Geometry: final body of the model. Coordinates: model frame, mm. A direction names the side the tool comes from. Round coordinates to 2 decimals unless told otherwise and drop trailing zeros. Loops run counter-clockwise (first coordinate to the right, second up) from the corner with the lowest first, then second, coordinate; pieces in that order, holes last. Notation, with made-up numbers: (-31.5, 73) - (-21.5, 73) arc R19 cw to (-21.5, 88) - close; hole circle Ø1 at (2.25, -20). An arc over 180 degrees is marked (long way). Use CSV: the item, a comma, the result in double quotes.
from build123d import *

# Parameters (mm, degrees)
F0_W     = 304.8
F0_H     = 508
F1_DEPTH = 45.72
F3_W     = 267.97
F3_H     = 480.06
F4_DEPTH = 88.9
F5_R     = 88.9
F6_DEPTH = 6.35
F7_R     = 15.24
F8_DEPTH = 12.7


with BuildPart() as f1:
    # F0 (on Top) → F1 (new body)
    with BuildSketch(Plane.XY):
        with Locations((-4.550833, 30.915228)):
            Rectangle(F0_W, F0_H)
    extrude(amount=F1_DEPTH)

    # F3 (on face) → F4 (join)
    with BuildSketch(Plane(origin=(0, 0, 0), x_dir=(1, 0, 0), z_dir=(0, 0, -1))):
        with Locations((-4.550833, -30.915228)):
            Rectangle(F3_W, F3_H)
    extrude(amount=F4_DEPTH)

    # F5 (on face) → F6 (cut)
    with BuildSketch(Plane.XY.offset(45.72)):
        with Locations((0, 157.915228)):
            Circle(F5_R)
        with Locations((0, -45.284772)):
            Circle(F5_R)
    extrude(amount=-F6_DEPTH, mode=Mode.SUBTRACT)

    # F7 (on face) → F8 (join)
    with BuildSketch(Plane.XY.offset(45.72)):
        with Locations((-42.650833, -185.567364)):
            Circle(F7_R)
        with Locations((33.549167, -185.567364)):
            Circle(F7_R)
    extrude(amount=F8_DEPTH)


solid = f1.part
Item 1: Mould query, pull axis Y, two halves, no side actions, for faces 1 (the cylindrical face through (-70.548, -99.379, 42.589)), 2 (the flat face through (-138.536, 34, -44)), 3 (the flat face through (-7, 284.915, 23)). Classes: released by +Y, released by -Y, zero draft, split by the parting line, or undercut.
Final values:
face 1,"undercut"
face 2,"zero draft"
face 3,"released by +Y"
Item 2: Section A-A on y = 254.5. Return the cut outline in (x, z).
Final values:
outline,"(-156.95, 0) - (-138.54, 0) - (-138.54, -88.9) - (129.43, -88.9) - (129.43, 0) - (147.85, 0) - (147.85, 45.72) - (-156.95, 45.72) - close"
Item 3: Pin query (flat end, axial travel): P1, Ø1, axis at y = 61.5, z = -57.5, coming from the +X side; P2, Ø8, axis at y = 207, z = -1, coming from the -X side; P3, Ø12, axis at x = -65, y = 171.5, coming from the +Z side; P4, Ø12, axis at x = 113.5, z = -43, coming from the -Y side. Return the tip coordinate at first contact, or that it passes through.
Final values:
P1,"stops at x = 129.43"
P2,"stops at x = -156.95"
P3,"stops at z = 39.37"
P4,"stops at y = -209.11"
Item 4: Section D-D on x = -76. Return the cut outline in (y, z), plus the area to 3 significant figures.
Final values:
outline,"(-223.08, 0) - (-209.11, 0) - (-209.11, -88.9) - (270.95, -88.9) - (270.95, 0) - (284.92, 0) - (284.92, 45.72) - (204.04, 45.72) - (204.04, 39.37) - (111.79, 39.37) - (111.79, 45.72) - (0.84, 45.72) - (0.84, 39.37) - (-91.41, 39.37) - (-91.41, 45.72) - (-223.08, 45.72) - close"
area,"64,700 mm²"
Item 5: Section C-C on z = -79.5. Return the cut outline in (x, y), plus the area to 3 significant figures.
Final values:
outline,"(-138.54, -209.11) - (129.43, -209.11) - (129.43, 270.95) - (-138.54, 270.95) - close"
area,"129,000 mm²"
Item 6: Reachability of faces 4 (the cylindrical face through (-45.955, -200.445, 51.981)), 5 (the flat face through (-6, 270.945, -44)), 6 (the flat face through (129.434, 34, -44)) from +Z, -Z, +X, -X, +Y, -Y: full face, straight path, thin tool, end or side. Return the list, or none.
Final values:
face 4,"+Z"
face 5,"-Z, +X, -X, +Y"
face 6,"-Z, +X, +Y, -Y"
Item 7: Section B-B on x = 0. Return the cut outline in (y, z).
Final values:
outline,"(-223.08, 0) - (-209.11, 0) - (-209.11, -88.9) - (270.95, -88.9) - (270.95, 0) - (284.92, 0) - (284.92, 45.72) - (246.82, 45.72) - (246.82, 39.37) - (69.02, 39.37) - (69.02, 45.72) - (43.62, 45.72) - (43.62, 39.37) - (-134.18, 39.37) - (-134.18, 45.72) - (-223.08, 45.72) - close"
Item 8: Material intervals for line 1 (Y direction, x = 0, z = 42.75); line 2 (Z direction, x = 100.5, y = -30.5); line 3 (Y direction, x = -80, z = -76), sorted ascending.
Final values:
line 1,"y = -223.08 to -134.18, 43.62 to 69.02, 246.82 to 284.92"
line 2,"z = -88.9 to 45.72"
line 3,"y = -209.11 to 270.95"
